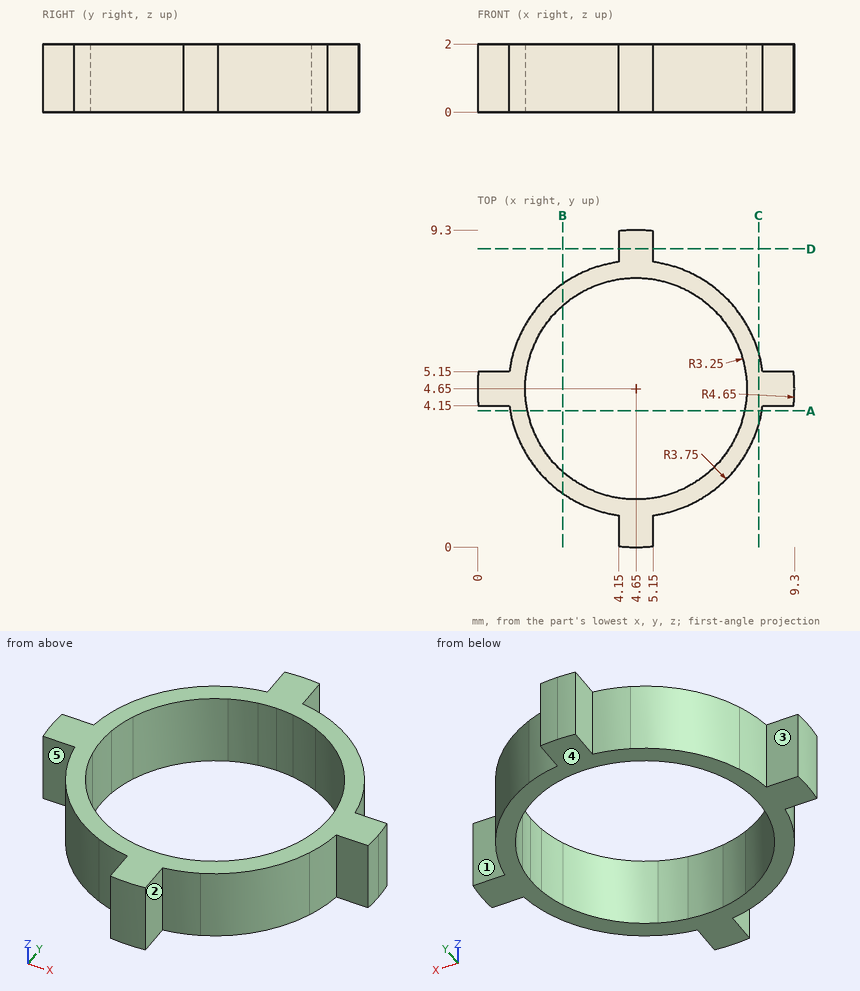
The figure shows three views and two pictorial views of one solid part (mm, origin at its lowest corner). Answer the questions. A direction names the side the tool comes from. Round coordinates to 2 decimals unless told otherwise and drop trailing zeros. Write each loop counter-clockwise with the first axis right and the second up, starting at its lowest first coordinate (ties: lowest second). Pieces come first, ordered by that corner, then holes. Notation, with made-up numbers: (-23, -5.75) - (32, -5.75) arc R21 ccw to (32, 22.25) - close; hole circle Ø1 at (51, 69.25). An arc over 180 degrees is marked (long way). Use one line per item in the form item = value. Start each with the question number.
Item 1: Find the intervals of material crossed by line 1 (X direction, y = 8.75, z = 1.35); line 2 (X direction, y = 6.5, z = 0.4); line 3 (Y direction, x = 6, z = 1.55), in increasing order. Write a range as [from, to].
Item 2: A cutting plane is placed at A-A (y = 4). Write down the section's boundary in (x, z), plus the area to 3 significant figures.
Item 3: A tool of negligible diameter and unlimited length cuts with its end or side. For the marked faces 1, 2, 3, 4 and 5, from which of +Z, -Z, +X, -X, +Y, -Y can it reach the whole face along a straight path? Write none if from no direction.
Item 4: A cutting plane is placed at B-B (x = 2.5). Write down the section's boundary in (y, z).
Item 5: A cutting plane is placed at D-D (y = 8.75). Write down the section's boundary in (x, z).
Item 6: Flat-ended cylindrical pins translate along their axes: pin 1 Ø0.5 at (y, z) = (0.5, 1) entering from +X; pin 2 Ø1 at (x, z) = (9, 0.5) entering from -Y; pin 3 Ø0.5 at (x, z) = (0.5, 1.5) entering from +Y. Find the tip coordinate at first contact, or state that the pin passes through.
Item 7: A cutting plane is placed at C-C (x = 8.25). Write down the section's boundary in (y, z).
The answers:
q1.line_1 = [4.15, 5.15]
q1.line_2 = [1.39, 1.98], [7.32, 7.91]
q1.line_3 = [1.15, 1.69], [7.61, 8.15]
q2.outline = (0.96, 0) - (1.47, 0) - (1.47, 2) - (0.96, 2) - close; (7.83, 0) - (8.34, 0) - (8.34, 2) - (7.83, 2) - close
q2.area = 2.04 mm^2
q3.face_1 = +Z, -Z, +X, +Y
q3.face_2 = +Z, -Z, +X, -Y
q3.face_3 = +Z, -Z, -X, +Y
q3.face_4 = -Z, +X, -X, +Y, -Y
q3.face_5 = +Z, -Z, -X, -Y
q4.outline = (1.58, 0) - (2.21, 0) - (2.21, 2) - (1.58, 2) - close; (7.09, 0) - (7.72, 0) - (7.72, 2) - (7.09, 2) - close
q5.outline = (4.15, 0) - (5.15, 0) - (5.15, 2) - (4.15, 2) - close
q6.pin_1 = 5.15
q6.pin_2 = 4.15
q6.pin_3 = 5.15
q7.outline = (3.6, 0) - (5.7, 0) - (5.7, 2) - (3.6, 2) - close
